Verification items for the finished model (mm, model axes). Coordinates: 2 decimals unless noted, no trailing zeros. Write each loop counter-clockwise with the first axis right and the second up, starting at its lowest first coordinate (ties: lowest second). Pieces come first, ordered by that corner, then holes. Notation, with made-up numbers: (77.25, 22) -> (86.25, 22) arc R23 ccw to (86.25, 41) -> close; hole circle Ø2 at (61, -25). An arc over 180 degrees is marked (long way). Write item = value, one per line. Start each with the question number.
(1) Section check D-D (x = 56.5). Record the cut outline in (y, z) (3 decimals).
(2) Mould release check, pull along Z, two halves, no side actions. Record for faces 1 (the face through (80.398, 1.565, -14.756)), 2 (the face through (98.953, 1.565, -89.715)), 3 (the face through (64, 3.175, -55)): released by +Z, released by -Z, zero draft, split by the parting line, or undercut.
(3) Section check B-B (z = -104.5). Record the cut outline in (x, y) (3 decimals).
(4) Gauge pin test, flat end, axial feed: pin 1 Ø1 at (y, z) = (1.5, -122.5) entering from +X. Record the tip position at first contact, or that the pin passes through.
(5) Section check C-C (y = 0.65). State how many separate pieces and enclosed holes the cut face has, plus the area to 3 significant figures.
(6) Material ranges on probe 1 along Z at (x, y) = (18.5, 0.55); probe 2 along X at (y, z) = (2.35, -81); probe 3 along X at (y, z) = (0.1, -107), recorded low to high. Write a range as [from, to].
(7) Section check A-A (x = 31.75). Record the cut outline in (y, z) (3 decimals).
```python
from build123d import *

# Parameters (mm, degrees)
SKETCH1_R           = 2.4257
BOSS_EXTRUDE1_DEPTH = 3.175
FILLET1_R           = 3.175
SKETCH2_R           = 4.3688
CUT_EXTRUDE1_DEPTH  = 214.780566999


with BuildPart() as part:
    # Sketch1 → Boss-Extrude1 (new body)
    with BuildSketch(Plane(origin=(0, 0, 0), x_dir=(1, 0, 0), z_dir=(0, 1, 0))):
        Polygon((0, 0), (0, 139.7), (38.1, 139.7), (161.789864335, 38.1), (161.789864335, 0), align=None)
        with Locations(Location((31.75, 15.875, 0), (0, 0, 270))):
            Circle(SKETCH1_R, mode=Mode.SUBTRACT)
        with Locations(Location((82.55, 15.875, 0), (0, 0, 270))):
            Circle(SKETCH1_R, mode=Mode.SUBTRACT)
        with Locations(Location((133.35, 15.875, 0), (0, 0, 270))):
            Circle(SKETCH1_R, mode=Mode.SUBTRACT)
        with Locations(Location((16.891, 53.975, 0), (0, 0, 270))):
            Circle(SKETCH1_R, mode=Mode.SUBTRACT)
        with Locations(Location((16.891, 79.375, 0), (0, 0, 270))):
            Circle(SKETCH1_R, mode=Mode.SUBTRACT)
        with Locations(Location((16.891, 104.775, 0), (0, 0, 270))):
            Circle(SKETCH1_R, mode=Mode.SUBTRACT)
        with Locations(Location((16.891, 130.175, 0), (0, 0, 270))):
            Circle(SKETCH1_R, mode=Mode.SUBTRACT)
    extrude(amount=BOSS_EXTRUDE1_DEPTH)

    # Fillet1
    fillet1_edges = [part.edges().sort_by_distance(p)[0] for p in [
        (0, 1.5875, 0),
        (0, 1.5875, -139.7),
        (38.1, 1.5875, -139.7),
        (161.789864335, 1.5875, -38.1),
        (161.789864335, 1.5875, 0),
    ]]
    fillet(fillet1_edges, radius=FILLET1_R)

    # Sketch2 → Cut-Extrude1 (cut, through all)
    with BuildSketch(Plane(origin=(0, 3.175, 0), x_dir=(1, 0, 0), z_dir=(0, 1, 0))):
        with Locations(Location((63.5, 63.5, 0), (0, 0, 270))):
            Circle(SKETCH2_R)
    extrude(amount=-CUT_EXTRUDE1_DEPTH, mode=Mode.SUBTRACT)


solid = part.part
```
Response:
q1.outline = (0, -124.586) -> (3.175, -124.586) -> (3.175, 0) -> (0, 0) -> close
q2.face_1 = undercut
q2.face_2 = released by -Z
q2.face_3 = zero draft
q3.outline = (0, 0) -> (14.481, 0) -> (14.481, 3.175) -> (0, 3.175) -> close; (19.301, 0) -> (80.953, 0) -> (80.953, 3.175) -> (19.301, 3.175) -> close
q4.pin_1 = 59.65
q5.separate_pieces = 1
q5.enclosed_holes = 8
q5.area = 16,100 mm2
q6.probe_1 = [-139.7, -131.99], [-128.36, -106.59], [-102.96, -81.19], [-77.56, -55.79], [-52.16, 0]
q6.probe_2 = [0, 15.09], [18.69, 109.56]
q6.probe_3 = [0, 15.92], [17.86, 77.91]
q7.outline = (0, -139.7) -> (3.175, -139.7) -> (3.175, -18.301) -> (0, -18.301) -> close; (0, -13.449) -> (3.175, -13.449) -> (3.175, 0) -> (0, 0) -> close
